```python
from build123d import *

# Parameters (mm, degrees)
SKETCH1_W           = 20
SKETCH1_H           = 20
BOSS_EXTRUDE1_DEPTH = 25
HOLE1_D             = 4
HOLE1_DEPTH         = 10
CUT_EXTRUDE1_DEPTH  = 18
CIRPATTERN1_COUNT   = 7
CIRPATTERN1_ANGLE   = 160


with BuildPart() as part:
    # Sketch1 → Boss-Extrude1 (new body)
    with BuildSketch(Plane.XY):
        with BuildLine():
            Line((-119, 0), (0, 0))
            ThreePointArc((0, 0), (-59.5, -59.5), (-119, 0))
        make_face()
        with Locations((-40, -25)):
            Rectangle(SKETCH1_W, SKETCH1_H, mode=Mode.SUBTRACT)
        with Locations((-79, -25)):
            Rectangle(SKETCH1_W, SKETCH1_H, mode=Mode.SUBTRACT)
    extrude(amount=BOSS_EXTRUDE1_DEPTH)

    # Hole1
    with Locations(Plane(origin=(-0.903938696, -10.332066571, 12.5), x_dir=(0.173648177667, 0.984807753012, 0), z_dir=(0.984807753012, -0.173648177667, 0))):
        with Locations((0, 0)):
            hole1 = Hole(HOLE1_D / 2, depth=HOLE1_DEPTH)

    # Sketch7 → Cut-Extrude1 (cut)
    with BuildSketch(Plane(origin=(0, 0, 0), x_dir=(-1, 0, 0), z_dir=(0, 0, -1))):
        Polygon((4.872912484, -4.047383041), (6.783042438, -14.880268324), (11.707081203, -14.012027436), (9.796951249, -3.179142153), align=None)
    cut_extrude1 = extrude(amount=-CUT_EXTRUDE1_DEPTH, mode=Mode.SUBTRACT)

    # CirPattern1: Hole1, Cut-Extrude1 ×7 about axis
    cirpattern1_axis = Axis((-59.5, 0, 0), (0, 0, -1))
    add([hole1.rotate(cirpattern1_axis, i * CIRPATTERN1_ANGLE / (CIRPATTERN1_COUNT - 1)) for i in range(1, CIRPATTERN1_COUNT)], mode=Mode.SUBTRACT)
    add([cut_extrude1.rotate(cirpattern1_axis, i * CIRPATTERN1_ANGLE / (CIRPATTERN1_COUNT - 1)) for i in range(1, CIRPATTERN1_COUNT)], mode=Mode.SUBTRACT)


solid = part.part
```
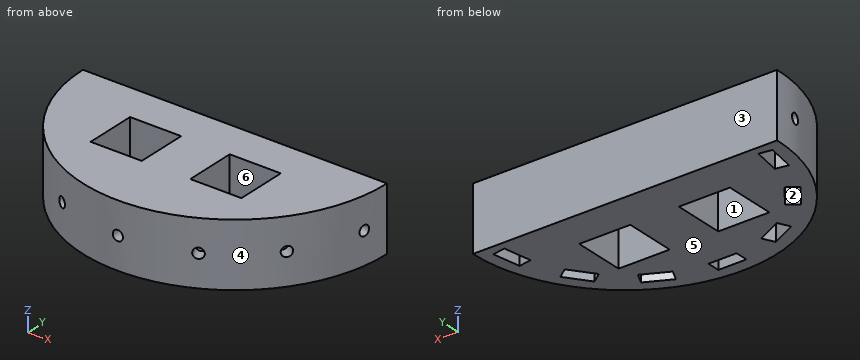
Here's how the part is built. I have some questions about the finished solid (model axes, mm). Face numbers are marked on the shaded views. A direction names the side the tool comes from. Give positions to 0.01 mm unless a question says otherwise; leave off trailing zeros. Loops run counter-clockwise (first coordinate to the right, second up) from the corner with the lowest first, then second, coordinate; pieces in that order, holes last. Notation, with made-up numbers: M -8.75,-29 L 21.25,-29 A13 cw 21.25,-17 Z; hole C -21,28.25 d7. An arc over 180 degrees is marked long. Use one line per item in the form item = value. Start each with the question number.
Q1. If we section it at A-A (x = -59.5): Write out the boundary of the cut face in (y, z).
Q2. If we section it at B-B (y = -26.5): Write out the boundary of the cut face in (x, z), then the cut area to 3 significant figures.
Q3. If we section it at C-C (z = 21): Write out the boundary of the cut face in (x, y), then the cut area to 3 significant figures.
Q4. I need wall thicknesses on line 1 along X through (y, z) = (-24, 13.5); line 2 along X through (y, z) = (-30.5, 1.75); line 3 along Z through (x, y) = (-59.5, -58). Which ranges of each line are inside material? Lowest first, please.
Q5. If we section it at D-D (x = -110.5): Write out the boundary of the cut face in (y, z).
Q6. Which directions (+Z, -Z, +X, -X, +Y, -Y) give clear straight access to the entire face, cutting with the end or side of a thin tool? Please do the marked faces 1, 2 and 3.
Q7. Thinking about a two-plate mould opening in X: for the marked faces 4, 5 and 6, which applies, +X half, -X half, draft (parallel to the pull), parting line (faces both ways), or undercut?
Q8. Will these pins go through, and if not, where does the flat tip stop? pin 1 Ø8 at (x, y) = (-45, -17) entering from -Z; pin 2 Ø6 at (x, z) = (-75, 12.5) entering from -Y; pin 3 Ø10 at (y, z) = (-25, 14.5) entering from +X; pin 4 Ø5 at (y, z) = (-19, 3.5) entering from +X.
Taken from the geometry:
q1.outline = M -59.5,0 L -54.5,0 L -54.5,10.5 L -59.5,10.5 Z; M -59.5,14.5 L -54.5,14.5 L -54.5,18 L -49.5,18 L -49.5,0 L 0,0 L 0,25 L -59.5,25 Z
q2.outline = M -112.77,0 L -104.31,0 L -104.31,18 L -101.48,18 L -101.48,0 L -89,0 L -89,25 L -112.77,25 Z; M -69,0 L -50,0 L -50,25 L -69,25 Z; M -30,0 L -17.52,0 L -17.52,18 L -14.69,18 L -14.69,0 L -6.23,0 L -6.23,25 L -30,25 Z
q2.area = 1,560 mm^2
q3.outline = M -119,0 A59.5 ccw 0,0 Z; hole M -89,-35 L -69,-35 L -69,-15 L -89,-15 Z; hole M -50,-35 L -30,-35 L -30,-15 L -50,-15 Z
q3.area = 4,760 mm^2
q4.line_1 = -113.94 to -89, -69 to -50, -30 to -5.06
q4.line_2 = -110.59 to -104.74, -98.5 to -89, -69 to -50, -30 to -20.5, -14.26 to -8.41
q4.line_3 = 0 to 10.5, 14.5 to 25
q5.outline = M -30.65,0 L -14.58,0 L -14.58,18 L -3.41,18 L -3.41,0 L 0,0 L 0,25 L -30.65,25 Z
q6.face_1 = +Z, -Z
q6.face_2 = -Z
q6.face_3 = +Z, -Z, +X, -X, +Y
q7.face_4 = parting line
q7.face_5 = draft
q7.face_6 = undercut
q8.pin_1 = 0
q8.pin_2 = -58.17
q8.pin_3 = -3.46
q8.pin_4 = -2.33
